```python
from build123d import *

# Parameters (mm, degrees)
F1_DEPTH = 8
F2_DEPTH = 18
F3_START = -18
F3_DEPTH = 32


with BuildPart() as f1:
    # F0 (on Front) → F1 (new body)
    with BuildSketch(Plane.XZ):
        with BuildLine():
            ThreePointArc((0, -11), (7.7781745931, -7.7781745931), (11, 0))
            ThreePointArc((11, 0), (10.1410640388, 4.2613167168), (7.6983963345, 7.8571428571))
            ThreePointArc((7.6983963345, 7.8571428571), (0, 9), (-7.6983963345, 7.8571428571))
            ThreePointArc((-7.6983963345, 7.8571428571), (-10.1840210975, -4.1576092031), (0, -11))
        make_face()
        with BuildLine():
            ThreePointArc((4.5, 0), (3.1819805153, -3.1819805153), (0, -4.5))
            ThreePointArc((0, -4.5), (-3.1819805153, 3.1819805153), (4.5, 0))
        make_face(mode=Mode.SUBTRACT)
        with BuildLine():
            ThreePointArc((-7.6983963345, 7.8571428571), (0, 9), (7.6983963345, 7.8571428571))
            ThreePointArc((7.6983963345, 7.8571428571), (0, 11), (-7.6983963345, 7.8571428571))
        make_face()
    extrude(amount=-F1_DEPTH)

    # F0 (on Front) → F2 (join)
    with BuildSketch(Plane.XZ):
        with BuildLine():
            ThreePointArc((0, -11), (7.7781745931, -7.7781745931), (11, 0))
            ThreePointArc((11, 0), (10.1410640388, 4.2613167168), (7.6983963345, 7.8571428571))
            ThreePointArc((7.6983963345, 7.8571428571), (0, 9), (-7.6983963345, 7.8571428571))
            ThreePointArc((-7.6983963345, 7.8571428571), (-10.1840210975, -4.1576092031), (0, -11))
        make_face()
        with BuildLine():
            ThreePointArc((4.5, 0), (3.1819805153, -3.1819805153), (0, -4.5))
            ThreePointArc((0, -4.5), (-3.1819805153, 3.1819805153), (4.5, 0))
        make_face(mode=Mode.SUBTRACT)
    extrude(amount=-F2_DEPTH)

    # F0 (on Front) → F3 (join)
    with BuildSketch(Plane.XZ.offset(F3_START)):
        with BuildLine():
            ThreePointArc((0, -11), (7.7781745931, -7.7781745931), (11, 0))
            ThreePointArc((11, 0), (10.1410640388, 4.2613167168), (7.6983963345, 7.8571428571))
            ThreePointArc((7.6983963345, 7.8571428571), (0, 9), (-7.6983963345, 7.8571428571))
            ThreePointArc((-7.6983963345, 7.8571428571), (-10.1840210975, -4.1576092031), (0, -11))
        make_face()
        with BuildLine():
            ThreePointArc((4.5, 0), (3.1819805153, -3.1819805153), (0, -4.5))
            ThreePointArc((0, -4.5), (-3.1819805153, 3.1819805153), (4.5, 0))
        make_face(mode=Mode.SUBTRACT)
        with BuildLine():
            ThreePointArc((-7.6983963345, 7.8571428571), (0, 9), (7.6983963345, 7.8571428571))
            ThreePointArc((7.6983963345, 7.8571428571), (0, 11), (-7.6983963345, 7.8571428571))
        make_face()
    extrude(amount=-F3_DEPTH)


solid = f1.part
```
CAD build for the part. Positions are in the model's coordinates, mm. A direction names the side the tool comes from. Give positions to 0.01 mm unless a question says otherwise; leave off trailing zeros. Order: outer loops, then holes, each group sorted by start corner. A loop starts at its lowest first (then second) coordinate and runs counter-clockwise, first axis right, second up.
(1) Mould opens along X. For faces 3 (the cylindrical face through (-4.496, 24.65, -0.198)), 4 (the flat face through (5, 50, 0)), 5 (the cylindrical face through (0, 25, -11)) say: released by +X, released by -X, zero draft, split by the parting line, or undercut.
(2) Flat gauge pins, fed straight in: pin 1 (5.5 mm diameter, centred on x = 0, z = 0, fed in from +Y); pin 2 (6 mm diameter, centred on y = 22.5, z = -6, fed in from -X); pin 3 (3 mm diameter, centred on x = -8.5, y = 9.5, fed in from +Z); pin 4 (1 mm diameter, centred on x = -8.5, y = 5.5, fed in from +Z). Where does each tip first touch, or does it go through?
(3) Saw through at C-C, the plane y = 19.5. Give the cut face in (x, z).
(4) Saw through at A-A, the plane z = 0. Give the cut face in (x, y), then the cut area to 3 significant figures.
(5) Saw through at D-D, the plane x = 5. Give the cut face in (y, z).
(6) Saw through at B-B, the plane x = 0. Give the cut face in (y, z), then the cut area to 3 significant figures.
(7) Tool access for faces 1 (the cylindrical face through (0, 13, 9)), 2 (the flat face through (5, 0, 0)): list every direction of +Z, -Z, +X, -X, +Y, -Y with a clear straight run to the whole face (end or side of a thin tool).
(8) Drill centre lines: L1, parallel to Z at x = 0, y = 18.5; L2, parallel to X at y = 45.5, z = 3.75; L3, parallel to Z at x = -1.75, y = 38. Where is each one in solid material? Low to high.
Results found:
1. face 3: undercut
1. face 4: zero draft
1. face 5: split by the parting line
2. pin 1: passes through
2. pin 2: stops at x = -10.58
2. pin 3: stops at z = 8.06
2. pin 4: stops at z = 7.55
3. outline: circle Ø22 at (0, 0); hole circle Ø9 at (0, 0)
4. outline: (-11, 0) - (-4.5, 0) - (-4.5, 50) - (-11, 50) - close; (4.5, 0) - (11, 0) - (11, 50) - (4.5, 50) - close
4. area: 650 mm2
5. outline: (0, -9.8) - (50, -9.8) - (50, 9.8) - (18, 9.8) - (18, 8.52) - (8, 8.52) - (8, 9.8) - (0, 9.8) - close
6. outline: (0, -11) - (50, -11) - (50, -4.5) - (0, -4.5) - close; (0, 4.5) - (50, 4.5) - (50, 11) - (18, 11) - (18, 9) - (8, 9) - (8, 11) - (0, 11) - close
6. area: 630 mm2
7. face 1: +Z
7. face 2: +Z, -Z, +X, -X, -Y
8. L1: z = -11 to -4.5, 4.5 to 11
8. L2: x = -10.34 to -2.49, 2.49 to 10.34
8. L3: z = -10.86 to -4.15, 4.15 to 10.86
